Here's how the part is built. I have some questions about the finished solid (model axes, mm). A direction names the side the tool comes from. Give positions to 0.01 mm unless a question says otherwise; leave off trailing zeros. Loops run counter-clockwise (first coordinate to the right, second up) from the corner with the lowest first, then second, coordinate; pieces in that order, holes last. Notation, with made-up numbers: (38.5, -9) -> (69.5, -9) arc R29 cw to (69.5, 26) -> close; hole circle Ø2 at (40.25, 5). An arc over 180 degrees is marked (long way). Answer in a Markdown table with one row per item. Add a question column.
Item 1: If we section it at D-D (y = -4.25): Write out the boundary of the cut face in (x, z).
Item 2: We'd pull the mould along X, two halves only. Please class faces 3 (the face through (9.93, -7.4, 6.53)), 4 (the face through (-5.75, 0.05, 3.04)), 5 (the face through (0, -8, 7)): released by +X, released by -X, zero draft, split by the parting line, or undercut.
Item 3: If we section it at B-B (z = 2.25): Write out the boundary of the cut face in (x, y).
Item 4: If we section it at A-A (x = -1.5): Write out the boundary of the cut face in (y, z), then the cut area to 4 significant figures.
Item 5: Which directions (+Z, -Z, +X, -X, +Y, -Y) give clear straight access to the entire face, cutting with the end or side of a thin tool? Please do faces 1 (the face through (2, 0, 0)), 2 (the face through (6.75, 0.05, 2.23)).
Item 6: If I drill on line 1 (X direction, y = 4.25, z = 7.75); line 2 (Y direction, x = -1.5, z = 2.75); line 3 (X direction, y = -4.25, z = 7), over which ranges is the centre line in solid material (lowest first)?
Item 7: For P1, Ø5.5, axis at x = 5.5, z = 7.25, coming from the -Y side, with a flat end and sliding along its axis, tell me the tip position at first contact or that it passes through.
Item 8: If we section it at C-C (x = -7): Write out the boundary of the cut face in (y, z).
```python
from build123d import *

# Parameters (mm, degrees)
SKETCH1_W                  = 21
SKETCH1_H                  = 16
BOSS_EXTRUDE1_DEPTH        = 11.5
F_10_CLEARANCE_HOLE1_D     = 5
F_12_CLEARANCE_HOLE1_D     = 6
F_2_CLEARANCE_HOLE1_REACH  = 19.507
F_2_CLEARANCE_HOLE1_BORE_R = 1.25
F_3_CLEARANCE_HOLE2_D      = 3
F_2_CLEARANCE_HOLE2_REACH  = 19.507
F_2_CLEARANCE_HOLE2_BORE_R = 1.25
CHAMFER2_SIZE              = 2
FILLET1_R                  = 2


with BuildPart() as part:
    # Sketch1 → Boss-Extrude1 (new body)
    with BuildSketch(Plane(origin=(0, 0, 0), x_dir=(-1, 0, 0), z_dir=(0, 0, -1))):
        Rectangle(SKETCH1_W, SKETCH1_H)
    extrude(amount=-BOSS_EXTRUDE1_DEPTH)

    # #10 Clearance Hole1 (through all)
    with Locations(Plane.XY.offset(11.5)):
        with Locations((-1.5, 0)):
            Hole(F_10_CLEARANCE_HOLE1_D / 2)

    # #12 Clearance Hole1 (through all)
    with Locations(Plane(origin=(0, 8, 0), x_dir=(1, 0, 0), z_dir=(0, 1, 0))):
        with Locations((5.5, -7.25)):
            Hole(F_12_CLEARANCE_HOLE1_D / 2)

    # #2 Clearance Hole1 bore → #2 Clearance Hole1 (cut, up to next)
    with BuildSketch(Plane(origin=(0, 0, 0), x_dir=(-1, 0, 0), z_dir=(0, 0, -1)), mode=Mode.PRIVATE) as f_2_clearance_hole1_sk1:
        with Locations((-5.5, 0)):
            Circle(F_2_CLEARANCE_HOLE1_BORE_R)
    f_2_clearance_hole1_tool1 = extrude(f_2_clearance_hole1_sk1.sketch, amount=-F_2_CLEARANCE_HOLE1_REACH, mode=Mode.PRIVATE) & part.part
    add(f_2_clearance_hole1_tool1.solids().sort_by_distance((5.5, 0, 0))[0], mode=Mode.SUBTRACT)

    # #3 Clearance Hole2 (through all)
    with Locations(Plane(origin=(0, -8, 0), x_dir=(-1, 0, 0), z_dir=(0, -1, 0))):
        with Locations((7, -7)):
            Hole(F_3_CLEARANCE_HOLE2_D / 2)

    # #2 Clearance Hole2 bore → #2 Clearance Hole2 (cut, up to next)
    with BuildSketch(Plane(origin=(0, 0, 0), x_dir=(-1, 0, 0), z_dir=(0, 0, -1)), mode=Mode.PRIVATE) as f_2_clearance_hole2_sk1:
        with Locations((7, 0)):
            Circle(F_2_CLEARANCE_HOLE2_BORE_R)
    f_2_clearance_hole2_tool1 = extrude(f_2_clearance_hole2_sk1.sketch, amount=-F_2_CLEARANCE_HOLE2_REACH, mode=Mode.PRIVATE) & part.part
    add(f_2_clearance_hole2_tool1.solids().sort_by_distance((-7, 0, 0))[0], mode=Mode.SUBTRACT)

    # Chamfer2
    chamfer2_edges = [part.edges().sort_by_distance(p)[0] for p in [
        (0, -8, 0),
        (10.5, 0, 0),
        (0, 8, 0),
        (-10.5, 0, 0),
    ]]
    chamfer(chamfer2_edges, length=CHAMFER2_SIZE)

    # Fillet1
    fillet1_edges = [part.edges().sort_by_distance(p)[0] for p in [
        (-10.5, -8, 6.75),
        (10.5, -8, 6.75),
        (10.5, 8, 6.75),
        (-10.5, 8, 6.75),
    ]]
    fillet(fillet1_edges, radius=FILLET1_R - 0.0001)  # a hair under: the kernel refuses the full size


solid = part.part
```
Recorded:
| question | item | result |
|---|---|---|
| 1 | outline | (-10.5, 2) -> (-8.5, 0) -> (8.5, 0) -> (10.5, 2) -> (10.5, 11.5) -> (-10.5, 11.5) -> close; hole circle Ø3 at (-7, 7); hole circle Ø6 at (5.5, 7.25) |
| 2 | face 3 | released by +X |
| 2 | face 4 | undercut |
| 2 | face 5 | zero draft |
| 3 | outline | (-10.5, -6) arc R2 ccw to (-8.5, -8) -> (8.5, -8) arc R2 ccw to (10.5, -6) -> (10.5, 6) arc R2 ccw to (8.5, 8) -> (-8.5, 8) arc R2 ccw to (-10.5, 6) -> close; hole circle Ø2.5 at (-7, 0); hole circle Ø5 at (-1.5, 0); hole circle Ø2.5 at (5.5, 0) |
| 4 | outline | (-8, 2) -> (-6, 0) -> (-2.5, 0) -> (-2.5, 11.5) -> (-8, 11.5) -> close; (2.5, 0) -> (6, 0) -> (8, 2) -> (8, 11.5) -> (2.5, 11.5) -> close |
| 4 | area | 122.5 mm^2 |
| 5 | face 1 | -Z, +X, -X, +Y, -Y |
| 5 | face 2 | -Z |
| 6 | line 1 | x = -10.5 to -8.3, -5.7 to 2.54, 8.46 to 10.5 |
| 6 | line 2 | y = -8 to -2.5, 2.5 to 8 |
| 6 | line 3 | x = -10.5 to -8.5, -5.5 to 2.51, 8.49 to 10.5 |
| 7 | P1 | passes through |
| 8 | outline | (-8, 2) -> (-6, 0) -> (-1.25, 0) -> (-1.25, 5.5) -> (-8, 5.5) -> close; (-8, 8.5) -> (8, 8.5) -> (8, 11.5) -> (-8, 11.5) -> close; (1.25, 0) -> (6, 0) -> (8, 2) -> (8, 5.5) -> (1.25, 5.5) -> close |
